Here's the drawing with two shaded views (mm, measured from the low corner). I have some questions. Give positions to 0.01 mm unless a question says otherwise; leave off trailing zeros. Write each loop counter-clockwise with the first axis right and the second up, starting at its lowest first coordinate (ties: lowest second). Pieces come first, ordered by that corner, then holes. Notation, with made-up numbers: (61, 80.5) -> (74, 80.5) arc R13 cw to (74, 88.5) -> close; hole circle Ø9 at (-26, 65.25). An arc over 180 degrees is marked (long way). One line per item, written item: value.
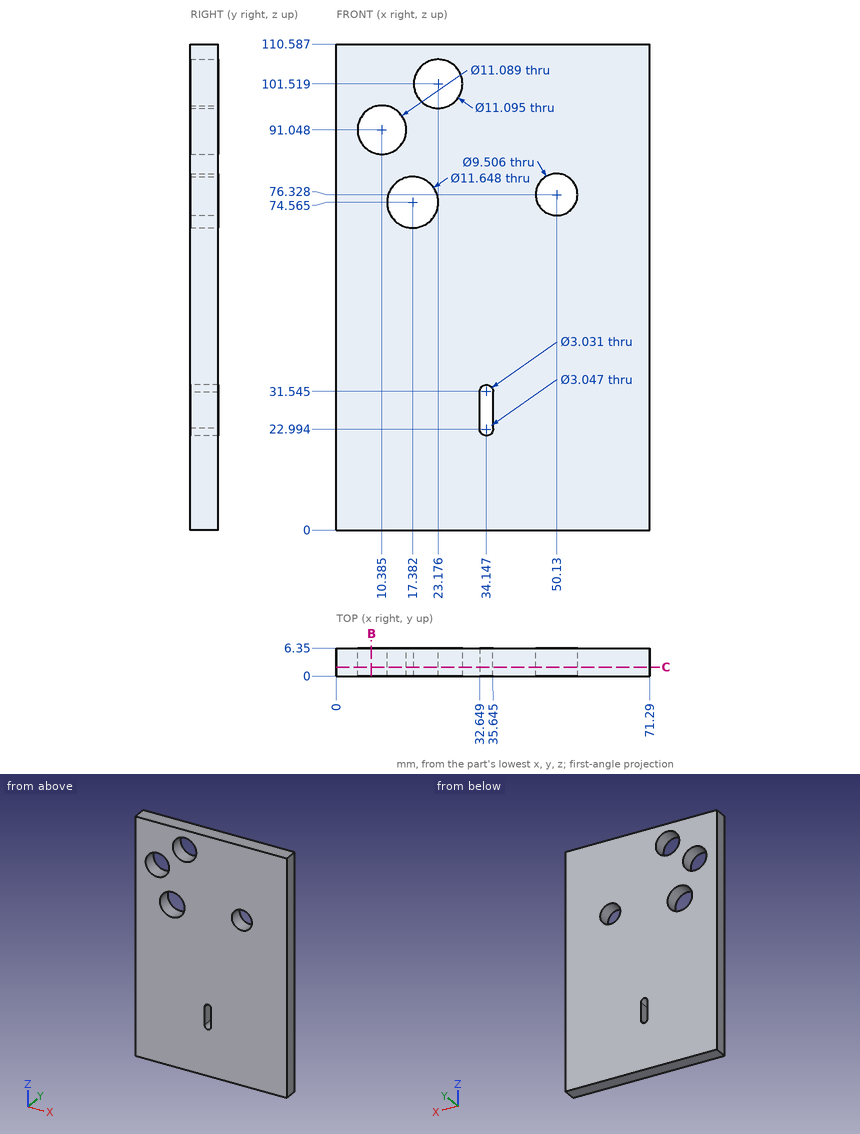
1) Will these pins go through, and if not, where does the flat tip stop? pin 1 (1 mm diameter, centred on x = 34, y = 2, fed in from -Z); pin 2 (2.5 mm diameter, centred on x = 34.15, z = 31.55, fed in from +Y).
Answer list:
pin 1: stops at z = 0
pin 2: passes through
2) If we section it at B-B (x = 8): Write out the boundary of the cut face in (y, z).
Answer list:
outline: (0, 0) -> (6.35, 0) -> (6.35, 86.04) -> (0, 86.04) -> close; (0, 96.05) -> (6.35, 96.05) -> (6.35, 110.59) -> (0, 110.59) -> close
3) I need wall thicknesses on L1, parallel to Z at x = 21, y = 3.25 (1 decimal); L2, parallel to X at y = 3, z = 78 (1 decimal); L3, parallel to Z at x = 22, y = 0.5 (1 decimal). Which ranges of each line are inside material? Lowest first, please.
Answer list:
L1: z = 0 to 70, 79.1 to 96.4, 106.6 to 110.6
L2: x = 0 to 12.7, 22.1 to 45.7, 54.6 to 71.3
L3: z = 0 to 71, 78.1 to 96.1, 106.9 to 110.6
4) If we section it at C-C (y = 2): State how many separate pieces and enclosed holes the cut face has, and give its area (3 significant figures).
Answer list:
separate pieces: 1
enclosed holes: 5
area: 7,480 mm^2
